Autodesk Inventor part; units mm, degrees
ref_plane "YZ Plane" through (0, 0, 0) normal (1, 0, 0) x (0, 1, 0)
ref_plane "XZ Plane" through (0, 0, 0) normal (0, 1, 0) x (-1, 0, 0)
ref_plane "XY Plane" through (0, 0, 0) normal (0, 0, 1) x (1, 0, 0)
sketch "草圖1" plane through (0, 0, 0) normal (0, 1, 0) x (-1, 0, 0)
  line L0 (4, 11.5) -> (-4, 11.5)
  line L1 (-4, -5.5) -> (4, -5.5)
  line L2 (-6, 2.5) -> (-6, -2.5)
  line L3 (6, -2.5) -> (6, 2.5)
  line L4 (6, 2.5) -> (4, 2.5)
  line L5 (-4, 2.5) -> (-6, 2.5)
  line L6 (4, -5.5) -> (4, -2.5)
  line L7 (-6, -2.5) -> (-4, -2.5)
  line L8 (4, -2.5) -> (6, -2.5)
  line L9 (-4, 11.5) -> (-4, 2.5)
  line L10 (-4, -2.5) -> (-4, -5.5)
  line L11 (0, 14.8546) -> (0, -17.157)
  line L12 (13.4413, 0) -> (-16.1444, 0)
  line L13 (4, 5.5) -> (0, 5.5)
  line L14 (0, 5.5) -> (0, 8.5)
  line L15 (0, 8.5) -> (4, 8.5)
  line L16 (4, 2.5) -> (4, 5.5)
  line L17 (4, 8.5) -> (4, 11.5)
  point P0 (0, 0)
  point P1 (-6, 0)
  point P2 (6, 0)
  dimension "d0" = 8
  dimension "d3" = 5
  dimension "d5" = 12
  dimension "d8" = 3
  dimension "d9" = 9
  dimension "d10" = 3
  dimension "d11" = 3
extrude "擠出1" add sketch "草圖1" along normal blind 3
properties part number "plug" material "木材 (楓木)"
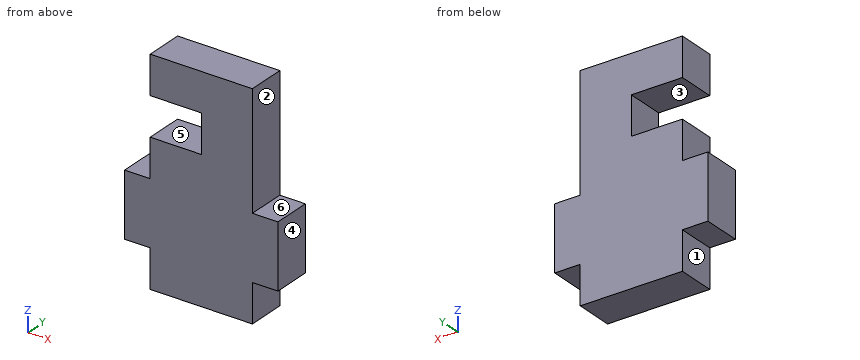
Input: part model. Units: mm. Frame: model coordinates. Face numbers are marked on the shaded views. A direction names the side the tool comes from. Coordinates: 2 decimals unless noted, no trailing zeros. Order: outer loops, then holes, each group sorted by start corner. A loop starts at its lowest first (then second) coordinate and runs counter-clockwise, first axis right, second up. Notation, with made-up numbers: M 8.25,68.5 L 62.25,68.5 A32 ccw 62.25,105.5 Z; hole C 52.5,-33 d1. An arc over 180 degrees is marked long. Answer in a Markdown table with one row per item.
(1) Draft query along Z for the marked faces 4, 5 and 6. Return one class per face: pulls with the +Z half, pulls with the -Z half, needs draft (parallel to the pull), parting line crosses it, or undercut.
Numbers:
| item | result |
|---|---|
| face 4 | needs draft |
| face 5 | undercut |
| face 6 | pulls with the +Z half |
(2) Section query A-A, the plane x = -1. Output: boundary loops of the cut face in (y, z).
Numbers:
| item | result |
|---|---|
| outline | M 0,-5.5 L 3,-5.5 L 3,5.5 L 0,5.5 Z; M 0,8.5 L 3,8.5 L 3,11.5 L 0,11.5 Z |
(3) Section query D-D, the plane x = -5. Output: boundary loops of the cut face in (y, z), plus the area to 3 significant figures.
Numbers:
| item | result |
|---|---|
| outline | M 0,-2.5 L 3,-2.5 L 3,2.5 L 0,2.5 Z |
| area | 15.0 mm^2 |
(4) Section query B-B, the plane y = 0.8. Output: boundary loops of the cut face in (x, z), plus the area to 3 significant figures.
Numbers:
| item | result |
|---|---|
| outline | M -6,-2.5 L -4,-2.5 L -4,-5.5 L 4,-5.5 L 4,-2.5 L 6,-2.5 L 6,2.5 L 4,2.5 L 4,11.5 L -4,11.5 L -4,8.5 L 0,8.5 L 0,5.5 L -4,5.5 L -4,2.5 L -6,2.5 Z |
| area | 144 mm^2 |
(5) Material intervals for line 1 (Z direction, x = -1, y = 0.75); line 2 (Z direction, x = 4.75, y = 1.65); line 3 (X direction, y = 1.8, z = -3.5), sorted ascending. Write a range as [from, to].
Numbers:
| item | result |
|---|---|
| line 1 | z = [-5.5, 5.5], [8.5, 11.5] |
| line 2 | z = [-2.5, 2.5] |
| line 3 | x = [-4, 4] |
(6) Section query C-C, the plane z = 6. Output: boundary loops of the cut face in (x, y).
Numbers:
| item | result |
|---|---|
| outline | M 0,0 L 4,0 L 4,3 L 0,3 Z |
(7) Access query for the marked faces 1, 2 and 3. Directions: +Z, -Z, +X, -X, +Y, -Y. A direction counts if a zero-diameter tool reaches every point of the face in a straight line with its end or side. Return the directions, or none.
Numbers:
| item | result |
|---|---|
| face 1 | -Z, -X, +Y, -Y |
| face 2 | +Z, +X, +Y, -Y |
| face 3 | -X, +Y, -Y |
(8) Contact query for flat-ended pins moving along their axis: pin 1 Ø0.9 at (y, z) = (1, 4.5) entering from -X; pin 2 Ø0.6 at (x, y) = (5, 2) entering from +Z; pin 3 Ø1.5 at (y, z) = (1.5, 8) entering from +X. Output: stop coordinate, or through.
Numbers:
| item | result |
|---|---|
| pin 1 | stops at x = -4 |
| pin 2 | stops at z = 2.5 |
| pin 3 | stops at x = 4 |
